The listing builds one solid part. Answer for the finished solid, in the listing's coordinates (mm). A direction names the side the tool comes from. Give positions to 0.01 mm unless a question says otherwise; leave off trailing zeros. Write each loop counter-clockwise with the first axis right and the second up, starting at its lowest first coordinate (ties: lowest second). Pieces come first, ordered by that corner, then holes. Notation, with made-up numbers: (68, 65) - (109, 65) arc R18 ccw to (109, 85) - close; hole circle Ø9 at (24.5, 59.25). An arc over 180 degrees is marked (long way). Return JSON: item names as keys, results as strings.
from build123d import *

# Parameters (mm, degrees)
F0_W      = 80
F0_H      = 70
F1_DEPTH  = 20
F2_W      = 60
F2_H      = 50
F3_DEPTH  = 10
F5_DEPTH  = 20.001
F6_W      = 10
F6_H      = 50
F7_DEPTH  = 60
F8_R      = 24.99999
F11_DEPTH = 10
F12_R     = 15
F13_DEPTH = 70.001


# Not quite as in the source:
# - a fillet or chamfer is up to 0.001 mm smaller than in the source, because OpenCascade refuses the exact size


with BuildPart() as f1:
    # F0 (on Top) → F1 (new body)
    with BuildSketch(Plane.XY):
        Rectangle(F0_W, F0_H)
    extrude(amount=F1_DEPTH)

    # F2 (on face) → F3 (cut)
    with BuildSketch(Plane(origin=(0, 0, 0), x_dir=(1, 0, 0), z_dir=(0, 0, -1))):
        Rectangle(F2_W, F2_H)
    extrude(amount=-F3_DEPTH, mode=Mode.SUBTRACT)

    # F4 (on face) → F5 (cut, through all)
    with BuildSketch(Plane.XY.offset(20)):
        with BuildLine():
            Line((7.5, -35), (7.5, -20))
            ThreePointArc((7.5, -20), (0, -12.5), (-7.5, -20))
            Line((-7.5, -20), (-7.5, -35))
            Line((-7.5, -35), (7.5, -35))
        make_face()
    extrude(amount=-F5_DEPTH, mode=Mode.SUBTRACT)

    # F6 (on face) → F7 (join)
    with BuildSketch(Plane.XY.offset(20)):
        with Locations((25, 0)):
            Rectangle(F6_W, F6_H)
    extrude(amount=F7_DEPTH)

    # F8 (radius 25 in the source; OpenCascade refuses exactly that, so slightly less here)
    f8_edges = [f1.edges().sort_by_distance(p)[0] for p in [
        (25, -25, 80),
        (25, 25, 80),
    ]]
    fillet(f8_edges, radius=F8_R)

    # F10 (on offset) → F11 (join)
    with BuildSketch(Plane(origin=(-30, 0, 0), x_dir=(0, -1, 0), z_dir=(-1, 0, 0))):
        with BuildLine():
            Line((15, 20), (15, 35))
            ThreePointArc((15, 35), (0, 80), (-15, 35))
            Line((-15, 35), (-15, 20))
            Line((-15, 20), (15, 20))
        make_face()
    extrude(amount=-F11_DEPTH)

    # F12 (on face) → F13 (cut, through all)
    with BuildSketch(Plane(origin=(-30, 0, 0), x_dir=(0, -1, 0), z_dir=(-1, 0, 0))):
        with Locations((0, 55)):
            Circle(F12_R)
    extrude(amount=-F13_DEPTH, mode=Mode.SUBTRACT)


solid = f1.part
Item 1: Consider L1, parallel to Z at x = 27.75, y = 0; L2, parallel to X at y = 7, z = 29.5; L3, parallel to Y at x = 29.5, z = 36.5. Determine where each line is inside the solid, lowest interval first.
Answer below:
{"L1": "z = 10 to 40, 70 to 80", "L2": "x = -30 to -20, 20 to 30", "L3": "y = -25 to 25"}
Item 2: The mould has two halves that part along X. Classify faces 5 (the face through (0, 0, 10)), 6 (the face through (30, 0, 36)), 7 (the face through (25.07, -17.871, 72.482)): +X half, -X half, draft (parallel to the pull), parting line (faces both ways), or undercut.
Answer below:
{"face 5": "undercut", "face 6": "+X half", "face 7": "draft"}
Item 3: A cutting plane is placed at B-B on z = 44. Determine the outline of the cut face in (x, y), then the cut area to 3 significant figures.
Answer below:
{"outline": "(-30, -22.45) - (-20, -22.45) - (-20, -10.2) - (-30, -10.2) - close; (-30, 10.2) - (-20, 10.2) - (-20, 22.45) - (-30, 22.45) - close; (20, -25) - (30, -25) - (30, -10.2) - (20, -10.2) - close; (20, 10.2) - (30, 10.2) - (30, 25) - (20, 25) - close", "area": "541 mm²"}
Item 4: For faces 1 (the face through (-25, -15, 27)), 2 (the face through (-25.07, -0.874, 79.985)), 3 (the face through (25, 25, 37)), 4 (the face through (-30, -11, 44)), determine the directions among +Z, -Z, +X, -X, +Y, -Y from which every point of the face is accessible in a straight line to the end or side of a thin tool.
Answer below:
{"face 1": "-X, -Y", "face 2": "-X", "face 3": "+Z, +X, -X, +Y", "face 4": "+Z, -X, +Y, -Y"}
Item 5: A cutting plane is placed at A-A on y = 8.5. Determine the outline of the cut face in (x, z).
Answer below:
{"outline": "(-40, 0) - (-30, 0) - (-30, 10) - (30, 10) - (30, 0) - (40, 0) - (40, 20) - (30, 20) - (30, 42.64) - (20, 42.64) - (20, 20) - (-20, 20) - (-20, 42.64) - (-30, 42.64) - (-30, 20) - (-40, 20) - close; (-30, 67.36) - (-20, 67.36) - (-20, 78.51) - (-30, 78.51) - close; (20, 67.36) - (30, 67.36) - (30, 78.51) - (20, 78.51) - close"}
Item 6: Flat-ended cylindrical pins translate along their axes: P1, Ø25, axis at x = 6, y = 11.5, coming from the -Z side; P2, Ø11, axis at x = 25, z = 40.5, coming from the +Y side; P3, Ø3, axis at x = -26.5, y = -2.5, coming from the +Z side. Find the tip coordinate at first contact, or state that the pin passes through.
Answer below:
{"P1": "stops at z = 10", "P2": "stops at y = 25", "P3": "stops at z = 79.98"}
Item 7: A cutting plane is placed at D-D on y = 18. Determine the outline of the cut face in (x, z).
Answer below:
{"outline": "(-40, 0) - (-30, 0) - (-30, 10) - (30, 10) - (30, 0) - (40, 0) - (40, 20) - (30, 20) - (30, 72.35) - (20, 72.35) - (20, 20) - (-40, 20) - close; (-30, 37.65) - (-20, 37.65) - (-20, 72.35) - (-30, 72.35) - close"}
